```python
from build123d import *


with BuildPart() as part:
    # Sketch1 → Revolve1 (revolve)
    with BuildSketch(Plane.XY, mode=Mode.PRIVATE) as revolve1_sk:
        with BuildLine():
            ThreePointArc((54.29249997, 5.6515), (51.042658326, 5.231868239), (48.006, 4.0005))
            Line((48.006, 4.0005), (-48.006, 4.0005))
            ThreePointArc((-48.006, 4.0005), (-51.042658379, 5.231868252), (-54.292500079, 5.6515))
            ThreePointArc((-54.292500079, 5.6515), (-57.542341698, 5.231868232), (-60.579, 4.0005))
            Line((-60.579, 4.0005), (-60.579, 0))
            Line((-60.579, 0), (48.006, 0))
            Line((48.006, 0), (60.579, 0))
            Line((60.579, 0), (60.579, 4.0005))
            ThreePointArc((60.579, 4.0005), (57.542341645, 5.231868246), (54.29249997, 5.6515))
        make_face()
    revolve(revolve1_sk.sketch.rotate(Axis((66.409028462, 0, 0), (1, 0, 0)), 180), axis=Axis((66.409028462, 0, 0), (1, 0, 0)))


solid = part.part
```
Check sheet for the modelled part. Datum: model origin and axes. Units: mm. Coordinates: 2 decimals unless noted, no trailing zeros. Loops run counter-clockwise (first coordinate to the right, second up) from the corner with the lowest first, then second, coordinate; pieces in that order, holes last.
1) Sectioned sample at A-A (x = -1). Record the boundary of the cut face in (y, z).
2) Release check for a two-part mould opening along X. For faces 1 (the face through (-0.7, 0.9, 3.9)), 2 (the face through (60.579, 0, 0)), 3 (the face through (-60.579, 0, 0)) record: released by +X, released by -X, zero draft, split by the parting line, or undercut.
3) Material ranges on probe 1 along X at (y, z) = (4.5, 1.75); probe 2 along X at (y, z) = (-2.25, 4.25); probe 3 along Y at (x, z) = (-5, 0.75), recorded low to high.
4) Gauge pin test, flat ends, axial feed: pin 1 (5 mm diameter, centred on x = 14, z = -1.5, fed in from -Y); pin 2 (4 mm diameter, centred on x = 23.5, y = 1.5, fed in from +Z); pin 3 (6 mm diameter, centred on x = -31, z = 3, fed in from +Y); pin 4 (2 mm diameter, centred on y = 2, z = -4.5, fed in from +X). Record the tip position at first contact, or that the pin passes through.
Check sheet entries:
1. outline: circle Ø8 at (0, 0)
2. face 1: undercut
2. face 2: released by +X
2. face 3: released by -X
3. probe 1: x = -58.81 to -49.78, 49.78 to 58.81
3. probe 2: x = -58.86 to -49.73, 49.73 to 58.86
3. probe 3: y = -3.93 to 3.93
4. pin 1: stops at y = -4
4. pin 2: stops at z = 4
4. pin 3: stops at y = 4
4. pin 4: stops at x = 60.58
